from build123d import *

# Parameters (mm, degrees)
SKETCH1_R           = 5
BOSS_EXTRUDE1_DEPTH = 3
SKETCH2_R           = 1.6
CUT_EXTRUDE1_DEPTH  = 303.669787062


with BuildPart() as part:
    # Sketch1 → Boss-Extrude1 (new body)
    with BuildSketch(Plane(origin=(0, 0, 0), x_dir=(1, 0, 0), z_dir=(0, 1, 0))):
        with BuildLine():
            Line((0, 40), (260, 40))
            ThreePointArc((260, 40), (300, 0), (260, -40))
            Line((260, -40), (0, -40))
            ThreePointArc((0, -40), (-40, 0), (0, 40))
        make_face()
        with Locations(Location((0, 0, 0), (0, 0, 270))):
            Circle(SKETCH1_R, mode=Mode.SUBTRACT)
        with BuildLine():
            Line((260, -5), (240, -5))
            ThreePointArc((240, -5), (235, 0), (240, 5))
            Line((240, 5), (260, 5))
            ThreePointArc((260, 5), (265, 0), (260, -5))
        make_face(mode=Mode.SUBTRACT)
    extrude(amount=BOSS_EXTRUDE1_DEPTH)

    # Sketch2 → Cut-Extrude1 (cut, through all)
    with BuildSketch(Plane(origin=(0, 3, 0), x_dir=(1, 0, 0), z_dir=(0, 1, 0))):
        with Locations(Location((78.5, 30, 0), (0, 0, 270))):
            Circle(SKETCH2_R)
        with Locations(Location((78.5, -30, 0), (0, 0, 270))):
            Circle(SKETCH2_R)
        with Locations(Location((181.5, -30, 0), (0, 0, 90))):
            Circle(SKETCH2_R)
        with Locations(Location((181.5, 30, 0), (0, 0, 90))):
            Circle(SKETCH2_R)
        with BuildLine():
            Line((80, 9.5), (80, -9.5))
            ThreePointArc((80, -9.5), (81.5, -11), (80, -12.5))
            Line((80, -12.5), (77, -12.5))
            ThreePointArc((77, -12.5), (75.5, -11), (77, -9.5))
            Line((77, -9.5), (77, 9.5))
            ThreePointArc((77, 9.5), (75.5, 11), (77, 12.5))
            Line((77, 12.5), (80, 12.5))
            ThreePointArc((80, 12.5), (81.5, 11), (80, 9.5))
        make_face()
        with BuildLine():
            Line((183, 12.5), (180, 12.5))
            ThreePointArc((180, 12.5), (178.5, 11), (180, 9.5))
            Line((180, 9.5), (180, -9.5))
            ThreePointArc((180, -9.5), (178.5, -11), (180, -12.5))
            Line((180, -12.5), (183, -12.5))
            ThreePointArc((183, -12.5), (184.5, -11), (183, -9.5))
            Line((183, -9.5), (183, 9.5))
            ThreePointArc((183, 9.5), (184.5, 11), (183, 12.5))
        make_face()
    extrude(amount=-CUT_EXTRUDE1_DEPTH, mode=Mode.SUBTRACT)


solid = part.part
The listing builds one solid part. Answer for the finished solid, in the listing's coordinates (mm). Give positions to 0.01 mm unless a question says otherwise; leave off trailing zeros. Loops run counter-clockwise (first coordinate to the right, second up) from the corner with the lowest first, then second, coordinate; pieces in that order, holes last. Notation, with made-up numbers: (18.25, 29) - (60.25, 29) arc R18 ccw to (60.25, 46) - close; hole circle Ø11 at (-25, -21.75). An arc over 180 degrees is marked (long way). Write each question's results on one line, items separated by ' | '.
1. For a pull along X with two mould halves and no side action, classify faces 1 (the face through (299.99, 1.48, -0.88)), 2 (the face through (-4.88, 1.48, -1.08)), 3 (the face through (132, 0, -1)) as +X half, -X half, draft (parallel to the pull), parting line (faces both ways), or undercut.
Resolved:
face 1: +X half | face 2: undercut | face 3: draft
2. Find section C-C, the plane z = -19.5. Write down the section's boundary in (x, y).
Resolved:
outline: (-34.92, 0) - (294.92, 0) - (294.92, 3) - (-34.92, 3) - close
3. Find section D-D, the plane z = 24.5. Write down the section's boundary in (x, y), then the cut area to 3 significant figures.
Resolved:
outline: (-31.62, 0) - (291.62, 0) - (291.62, 3) - (-31.62, 3) - close | area: 970 mm^2
4. Consider probe 1 along Z at (x, y) = (78.5, 1.25); probe 2 along X at (y, z) = (1.7, 0); probe 3 along X at (y, z) = (0.7, 30). Determine where each line is inside the solid, lowest interval first. Write a range as from..to.
Resolved:
probe 1: z = -40..-31.6, -28.4..-12.5, 12.5..28.4, 31.6..40 | probe 2: x = -40..-5, 5..77, 80..180, 183..235, 265..300 | probe 3: x = -26.46..76.9, 80.1..179.9, 183.1..286.46
5. Flat-ended cylindrical pins translate along their axes: P1, Ø5, axis at x = 78.5, z = 30, coming from the -Y side; P2, Ø2.5, axis at x = 181.5, z = 30, coming from the -Y side. Find the tip coordinate at first contact, or state that the pin passes through.
Resolved:
P1: stops at y = 0 | P2: passes through
6. Find section B-B, the plane z = 0. Write down the section's boundary in (x, y).
Resolved:
outline: (-40, 0) - (-5, 0) - (-5, 3) - (-40, 3) - close; (5, 0) - (77, 0) - (77, 3) - (5, 3) - close; (80, 0) - (180, 0) - (180, 3) - (80, 3) - close; (183, 0) - (235, 0) - (235, 3) - (183, 3) - close; (265, 0) - (300, 0) - (300, 3) - (265, 3) - close
7. Find section A-A, the plane y = 2.3. Count the separate pieces of the cut face and the enclosed holes in it, then the cut area to 3 significant figures.
Resolved:
separate pieces: 1 | enclosed holes: 8 | area: 25,300 mm^2
